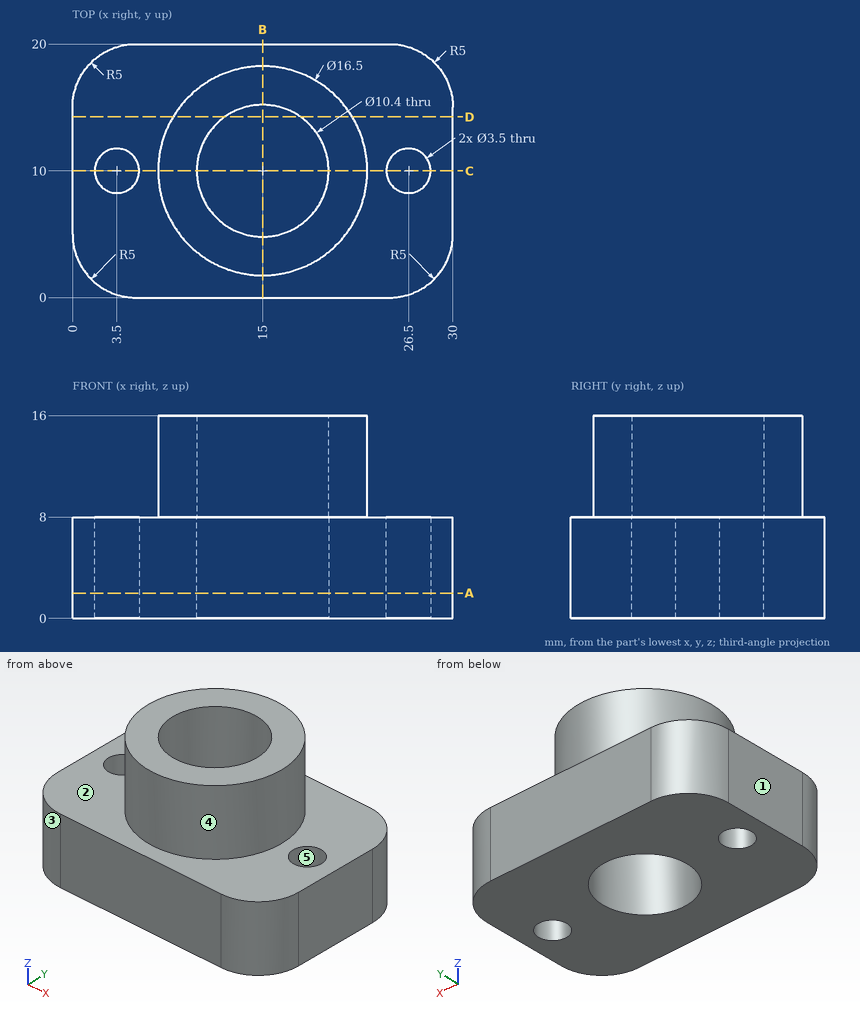
Print and shaded views of the part. All mm, measured from the part's lowest x, y and z. A direction names the side the tool comes from. Round coordinates to 2 decimals unless told otherwise and drop trailing zeros. Write each loop counter-clockwise with the first axis right and the second up, starting at its lowest first coordinate (ties: lowest second). Pieces come first, ordered by that corner, then holes. Notation, with made-up numbers: (87.5, 86) -> (138.5, 86) arc R33 cw to (138.5, 117) -> close; hole circle Ø2 at (69.25, -37). An arc over 180 degrees is marked (long way). Answer in a Markdown table with one row per item. Add a question column.
Item 1: Which spindle directions (+Z, -Z, +X, -X, +Y, -Y) get a long thin tool onto all of the face, cutting with end or side? Do the marked faces 1 and 2. Say none if no direction does.
Item 2: Mould opens along Y. For the marked faces 3, 4 and 5 say: pulls with the +Y half, pulls with the -Y half, needs draft (parallel to the pull), parting line crosses it, or undercut.
Item 3: Saw through at B-B, the plane x = 15. Write the cut outline in (y, z), then the cut area to 3 significant figures.
Item 4: Saw through at D-D, the plane y = 14.25. Write the cut outline in (x, z).
Item 5: Drill centre lines: line 1 (Z direction, x = 4.5, y = 12.25); line 2 (Y direction, x = 15.25, z = 12.25); line 3 (Y direction, x = 26.5, z = 5.75). Where is each one in solid material? Low to high. Write a range as from..to.
Item 6: Drop flat-ended pins along their axis: pin 1 Ø4 at (x, y) = (26.5, 10) entering from +Z; pin 2 Ø9.5 at (x, y) = (15, 10) entering from -Z; pin 3 Ø4 at (x, y) = (11.5, 18) entering from -Z; pin 4 Ø3 at (x, z) = (14.5, 11) entering from -Y. Give the stop position or say it passes through.
Item 7: Saw through at C-C, the plane y = 10. Write the cut outline in (x, z), then the cut area to 3 significant figures.
Item 8: Saw through at A-A, the plane z = 2. Write the cut outline in (x, y).
Findings below:
| question | item | result |
|---|---|---|
| 1 | face 1 | +Z, -Z, -X, +Y, -Y |
| 1 | face 2 | +Z |
| 2 | face 3 | pulls with the -Y half |
| 2 | face 4 | parting line crosses it |
| 2 | face 5 | undercut |
| 3 | outline | (0, 0) -> (4.8, 0) -> (4.8, 16) -> (1.75, 16) -> (1.75, 8) -> (0, 8) -> close; (15.2, 0) -> (20, 0) -> (20, 8) -> (18.25, 8) -> (18.25, 16) -> (15.2, 16) -> close |
| 3 | area | 126 mm^2 |
| 4 | outline | (0, 0) -> (12, 0) -> (12, 16) -> (7.93, 16) -> (7.93, 8) -> (0, 8) -> close; (18, 0) -> (30, 0) -> (30, 8) -> (22.07, 8) -> (22.07, 16) -> (18, 16) -> close |
| 5 | line 1 | z = 0..8 |
| 5 | line 2 | y = 1.75..4.81, 15.19..18.25 |
| 5 | line 3 | y = 0.23..8.25, 11.75..19.77 |
| 6 | pin 1 | stops at z = 8 |
| 6 | pin 2 | passes through |
| 6 | pin 3 | stops at z = 0 |
| 6 | pin 4 | stops at y = 1.75 |
| 7 | outline | (0, 0) -> (1.75, 0) -> (1.75, 8) -> (0, 8) -> close; (5.25, 0) -> (9.8, 0) -> (9.8, 16) -> (6.75, 16) -> (6.75, 8) -> (5.25, 8) -> close; (20.2, 0) -> (24.75, 0) -> (24.75, 8) -> (23.25, 8) -> (23.25, 16) -> (20.2, 16) -> close; (28.25, 0) -> (30, 0) -> (30, 8) -> (28.25, 8) -> close |
| 7 | area | 150 mm^2 |
| 8 | outline | (0, 5) arc R5 ccw to (5, 0) -> (25, 0) arc R5 ccw to (30, 5) -> (30, 15) arc R5 ccw to (25, 20) -> (5, 20) arc R5 ccw to (0, 15) -> close; hole circle Ø3.5 at (3.5, 10); hole circle Ø10.4 at (15, 10); hole circle Ø3.5 at (26.5, 10) |
